```python
from build123d import *

# Parameters (mm, degrees)
BOSS_EXTRUDE1_DEPTH = 7.62


with BuildPart() as part:
    # Sketch1 → Boss-Extrude1 (new body)
    with BuildSketch(Plane(origin=(0, 0, 0), x_dir=(1, 0, 0), z_dir=(0, 1, 0))):
        with BuildLine():
            Line((-13.883314172, 5.08), (68.666685828, 5.08))
            ThreePointArc((68.666685828, 5.08), (87.62550393, 0), (68.666685828, -5.08))
            Line((68.666685828, -5.08), (-13.883314172, -5.08))
            ThreePointArc((-13.883314172, -5.08), (-19.3763981, -9.60717032), (-26.492132275, -9.418572079))
            Line((-26.492132275, -9.418572079), (-26.492132275, -6.35))
            Line((-26.492132275, -6.35), (-19.998306484, -6.35))
            Line((-19.998306484, -6.35), (-16.332132275, 0))
            Line((-16.332132275, 0), (-19.998306484, 6.35))
            Line((-19.998306484, 6.35), (-26.492132275, 6.35))
            Line((-26.492132275, 6.35), (-26.492132275, 9.418572079))
            ThreePointArc((-26.492132275, 9.418572079), (-19.3763981, 9.60717032), (-13.883314172, 5.08))
        make_face()
        Polygon((70.133155511, 0), (73.799329721, -6.35), (81.131678139, -6.35), (84.797852349, 0), (81.131678139, 6.35), (73.799329721, 6.35), align=None, mode=Mode.SUBTRACT)
    extrude(amount=BOSS_EXTRUDE1_DEPTH)


solid = part.part
```
CAD build for the part. Positions are in the model's coordinates, mm. A direction names the side the tool comes from. Round coordinates to 2 decimals unless told otherwise and drop trailing zeros. Write each loop counter-clockwise with the first axis right and the second up, starting at its lowest first coordinate (ties: lowest second). Pieces come first, ordered by that corner, then holes. Notation, with made-up numbers: (-23.5, 48) -> (21.5, 48) arc R15 cw to (21.5, 76) -> close; hole circle Ø7 at (68.25, 43). An arc over 180 degrees is marked (long way). Answer in a Markdown table with one row per item. Add a question column.
Item 1: Which spindle directions (+Z, -Z, +X, -X, +Y, -Y) get a long thin tool onto all of the face, cutting with end or side? Do faces 1 (the face through (-18.19, 3.76, 3.22)), 2 (the face through (71.99, 3.76, -3.22)), 3 (the face through (28, 4, 5.08)), 4 (the face through (31, 0, 0)). Say none if no direction does.
Item 2: Drop flat-ended pins along their axis: pin 1 Ø4 at (x, y) = (17.5, 5) entering from -Z; pin 2 Ø2 at (x, y) = (76, 3) entering from +Z; pin 3 Ø2.5 at (x, y) = (19.5, 4) entering from +Z. Give the stop position or say it passes through.
Item 3: Saw through at C-C, the plane z = -3. Write the cut outline in (x, y).
Item 4: Saw through at B-B, the plane z = 2.75. Write the cut outline in (x, y).
Item 5: Saw through at D-D, the plane x = 31.5. Write the cut outline in (y, z), then the cut area to 3 significant figures.
Item 6: Drill centre lines: line 1 (X direction, y = 1.25, z = -5.5); line 2 (X direction, y = 5.25, z = -5.75); line 3 (Z direction, x = 50, y = 6). Where is each one in solid material? Low to high. Write a range as from..to.
Item 7: Saw through at A-A, the plane y = 6.5. Write the cut outline in (x, z), then the cut area to 3 significant figures.
Item 8: Mould opens along Z. For faces 5 (the face through (87.62, 3.76, -0.37)), 6 (the face through (82.99, 3.76, -3.13)), 7 (the face through (27, 4, -5.08)), 8 (the face through (-23, 4, 6.35)) say: pulls with the +Z half, pulls with the -Z half, needs draft (parallel to the pull), parting line crosses it, or undercut.
Findings below:
| question | item | result |
|---|---|---|
| 1 | face 1 | -X, +Y, -Y |
| 1 | face 2 | +Y, -Y |
| 1 | face 3 | +Z, +Y, -Y |
| 1 | face 4 | +Z, -Z, +X, -X, -Y |
| 2 | pin 1 | stops at z = -5.08 |
| 2 | pin 2 | stops at z = 10.15 |
| 2 | pin 3 | stops at z = 5.08 |
| 3 | outline | (-18.06, 0) -> (71.87, 0) -> (71.87, 7.62) -> (-18.06, 7.62) -> close; (83.07, 0) -> (87.17, 0) -> (87.17, 7.62) -> (83.07, 7.62) -> close |
| 4 | outline | (-17.92, 0) -> (71.72, 0) -> (71.72, 7.62) -> (-17.92, 7.62) -> close; (83.21, 0) -> (87.25, 0) -> (87.25, 7.62) -> (83.21, 7.62) -> close |
| 5 | outline | (0, -5.08) -> (7.62, -5.08) -> (7.62, 5.08) -> (0, 5.08) -> close |
| 5 | area | 77.4 mm^2 |
| 6 | line 1 | x = -19.51..-14.14, 68.92..73.31, 81.62..86.01 |
| 6 | line 2 | x = -19.65..-14.31, 69.09..73.45, 81.48..85.84 |
| 6 | line 3 | z = -5.08..5.08 |
| 7 | outline | (-26.49, -9.42) arc R10.16 ccw to (-13.88, -5.08) -> (68.67, -5.08) arc R10.16 ccw (long way) to (68.67, 5.08) -> (-13.88, 5.08) arc R10.16 ccw to (-26.49, 9.42) -> (-26.49, 6.35) -> (-20, 6.35) -> (-16.33, 0) -> (-20, -6.35) -> (-26.49, -6.35) -> close; hole (70.13, 0) -> (73.8, -6.35) -> (81.13, -6.35) -> (84.8, 0) -> (81.13, 6.35) -> (73.8, 6.35) -> close |
| 7 | area | 1,140 mm^2 |
| 8 | face 5 | parting line crosses it |
| 8 | face 6 | undercut |
| 8 | face 7 | pulls with the -Z half |
| 8 | face 8 | undercut |
